```python
from build123d import *

# Parameters (mm, degrees)
BASE_EXTRUDE_DEPTH      = 4.04
BASE_EXTRUDE_DEPTH_BACK = 1.5
SKETCH1_W               = 6.6
SKETCH1_H               = 3.18
SKETCH2_OUTSIDE_W       = 10.436
SKETCH2_OUTSIDE_H       = 7.016
CUT_EXTRUDE1_DEPTH      = 10.990985937
SKETCH3_OUTSIDE_W       = 9.376
SKETCH3_OUTSIDE_H       = 7.016
CUT_EXTRUDE2_DEPTH      = 9.857635125
SKETCH5_W               = 1.63
SKETCH5_H               = 0.38
BOSS_EXTRUDE3_DEPTH     = 0.7
SKETCH6_W               = 0.38
SKETCH6_H               = 1.63
BOSS_EXTRUDE4_DEPTH     = 2.53
SKETCH4_W               = 0.38
SKETCH4_H               = 0.56
BOSS_EXTRUDE5_DEPTH     = 3.28
CUT_EXTRUDE5_DEPTH      = 0.38
FILLET1_R               = 0.49
FILLET2_R               = 0.11
FILLET1_OF_MIRROR1_R    = 0.49
FILLET2_OF_MIRROR1_R    = 0.11
SKETCH10_R              = 0.75
CUT_EXTRUDE6_DEPTH      = 0.7


# Read off the part's stored shape, not the designer's step: Mirror2
with BuildPart() as part:
    # Sketch1 → Base-Extrude (new, two sides: drawn at the far end of the back side and taken through both)
    with BuildSketch(Plane.XY.offset(-BASE_EXTRUDE_DEPTH_BACK)):
        with Locations((3.81, 2.72)):
            Rectangle(SKETCH1_W, SKETCH1_H)
    extrude(amount=BASE_EXTRUDE_DEPTH + BASE_EXTRUDE_DEPTH_BACK)

    # Sketch2 outside → Cut-Extrude1 (cut, through all)
    with BuildSketch(Plane.XY.offset(4.04)):
        with Locations((3.81, 2.72)):
            Rectangle(SKETCH2_OUTSIDE_W, SKETCH2_OUTSIDE_H)
        with BuildLine():
            Line((0.51, 2.91), (0.679431307, 3.748623606))
            ThreePointArc((0.679431307, 3.748623606), (0.922305346, 4.151773257), (1.365567952, 4.31))
            Line((1.365567952, 4.31), (6.254432048, 4.31))
            ThreePointArc((6.254432048, 4.31), (6.697694654, 4.151773257), (6.940568693, 3.748623606))
            Line((6.940568693, 3.748623606), (7.11, 2.91))
            Line((7.11, 2.91), (7.11, 2.53))
            Line((7.11, 2.53), (6.940568693, 1.691376394))
            ThreePointArc((6.940568693, 1.691376394), (6.697694654, 1.288226743), (6.254432048, 1.13))
            Line((6.254432048, 1.13), (1.365567952, 1.13))
            ThreePointArc((1.365567952, 1.13), (0.922305346, 1.288226743), (0.679431307, 1.691376394))
            Line((0.679431307, 1.691376394), (0.51, 2.53))
            Line((0.51, 2.53), (0.51, 2.91))
        make_face(mode=Mode.SUBTRACT)
    extrude(amount=-CUT_EXTRUDE1_DEPTH, mode=Mode.SUBTRACT)

    # Sketch3 outside → Cut-Extrude2 (cut, through all)
    with BuildSketch(Plane(origin=(7.11, 0, 0), x_dir=(0, 0, -1), z_dir=(1, 0, 0))):
        with Locations((-1.27, 2.72)):
            Rectangle(SKETCH3_OUTSIDE_W, SKETCH3_OUTSIDE_H)
        Polygon((1.5, 2.91), (1.134316679, 4.72), (-3.674316679, 4.72), (-4.04, 2.91), (-4.04, 2.53), (-3.674316679, 0.72), (1.134316679, 0.72), (1.5, 2.53), align=None, mode=Mode.SUBTRACT)
    extrude(amount=-CUT_EXTRUDE2_DEPTH, mode=Mode.SUBTRACT)

    # Sketch5 → Boss-Extrude3 (add)
    with BuildSketch(Plane.ZY.offset(-0.51)):
        with Locations((0, 2.72)):
            Rectangle(SKETCH5_W, SKETCH5_H)
    boss_extrude3 = extrude(amount=BOSS_EXTRUDE3_DEPTH)

    # Sketch6 → Boss-Extrude4 (add)
    with BuildSketch(Plane.XZ.offset(-2.53)):
        Rectangle(SKETCH6_W, SKETCH6_H)
    boss_extrude4 = extrude(amount=BOSS_EXTRUDE4_DEPTH)

    # Sketch4 → Boss-Extrude5 (add)
    with BuildSketch(Plane(origin=(0, 0, 0), x_dir=(1, 0, 0), z_dir=(0, 1, 0))):
        Rectangle(SKETCH4_W, SKETCH4_H)
    boss_extrude5 = extrude(amount=-BOSS_EXTRUDE5_DEPTH)

    # Sketch7 → Cut-Extrude5 (cut)
    with BuildSketch(Plane.ZY.offset(0.19)):
        Polygon((0.815, 1.52), (0.55, 0.05), (0.28, 0), (0.28, -3.15), (0.15, -3.28), (-0.15, -3.28), (-0.28, -3.15), (-0.28, 0), (-0.55, 0.05), (-0.815, 1.52), (-0.815, -3.78), (0.815, -3.78), align=None)
    cut_extrude5 = extrude(amount=-CUT_EXTRUDE5_DEPTH, mode=Mode.SUBTRACT)

    # Fillet1
    fillet1_edges = [part.edges().sort_by_distance(p)[0] for p in [
        (-0.19, 2.91, 0),
    ]]
    fillet(fillet1_edges, radius=FILLET1_R)

    # Fillet2
    fillet2_edges = [part.edges().sort_by_distance(p)[0] for p in [
        (0.19, 2.53, 0),
    ]]
    fillet(fillet2_edges, radius=FILLET2_R)

    # Mirror1: Boss-Extrude3, Boss-Extrude4, Boss-Extrude5, Cut-Extrude5 across plane
    add(boss_extrude3.mirror(Plane.ZY.offset(-3.81)))
    add(boss_extrude4.mirror(Plane.ZY.offset(-3.81)))
    add(boss_extrude5.mirror(Plane.ZY.offset(-3.81)))
    add(cut_extrude5.mirror(Plane.ZY.offset(-3.81)), mode=Mode.SUBTRACT)

    # Fillet1 of Mirror1
    fillet1_of_mirror1_edges = [part.edges().sort_by_distance(p)[0] for p in [
        (7.81, 2.91, 0),
    ]]
    fillet(fillet1_of_mirror1_edges, radius=FILLET1_OF_MIRROR1_R)

    # Fillet2 of Mirror1
    fillet2_of_mirror1_edges = [part.edges().sort_by_distance(p)[0] for p in [
        (7.43, 2.53, 0),
    ]]
    fillet(fillet2_of_mirror1_edges, radius=FILLET2_OF_MIRROR1_R)

    # Mirror2: part across plane


with BuildPart() as part_1:
    add(part.part)
    add(part.part.mirror(Plane(origin=(0, 0, 1.27), x_dir=(1, 0, 0), z_dir=(0, 0, -1))))

    # Sketch9 → Cut-Revolve1 (revolve, cut)
    with BuildSketch(Plane.XY):
        with BuildLine():
            Line((2.980337349, 4.31), (2.230337349, 4.31))
            Line((2.230337349, 4.31), (2.230337349, 3.56))
            ThreePointArc((2.230337349, 3.56), (2.760667435, 3.779669914), (2.980337349, 4.31))
        make_face()
    revolve(axis=Axis((2.230337349, 5.149947403, 0), (0, -1, 0)), mode=Mode.SUBTRACT)

    # Sketch10 → Cut-Extrude6 (cut)
    with BuildSketch(Plane(origin=(0, 4.31, 0), x_dir=(-1, 0, 0), z_dir=(0, 1, 0))):
        with Locations((-3.81, -1.5)):
            Circle(SKETCH10_R)
    extrude(amount=-CUT_EXTRUDE6_DEPTH, mode=Mode.SUBTRACT)


solid = part_1.part
```
Part model, mm, in its own coordinate system. A direction names the side the tool comes from. Round coordinates to 2 decimals unless told otherwise and drop trailing zeros. Order: outer loops, then holes, each group sorted by start corner. A loop starts at its lowest first (then second) coordinate and runs counter-clockwise, first axis right, second up. Notation, with made-up numbers: M 5,57.25 L 34,57.25 A3 ccw 34,62.25 Z; hole C -1,-8.5 d8. An arc over 180 degrees is marked long. Answer in a Markdown table with one row per item. Add a question column.
Q1. Cut at B-B on x = 5. Give the cut face in (y, z).
Q2. Pin check, flat tips, straight feed: pin 1 (3 mm diameter, centred on x = 2.5, z = 0, fed in from -Y); pin 2 (0.6 mm diameter, centred on x = 7.5, y = 2, fed in from +Z) (3 decimals). Stop position of each tip, or through.
Q3. Cut at D-D on x = 2.5. Give the cut face in (y, z), and give its area (3 significant figures).
Q4. Mould opens along X. For faces 1 (the face through (4, 4.31, 1)), 2 (the face through (7.026, 2.117, 1.309)), 3 (the face through (0.594, 3.323, 1.309)) say: +X half, -X half, draft (parallel to the pull), parting line (faces both ways), or undercut.
Q5. Cut at A-A on y = -1.75. Give the cut face in (x, z), and give its area (3 significant figures).
Q6. 3-axis set-ups, long thin cutter, end or side, ignore diameter. For faces 4 (the face through (0.19, 0.2, 2.6)), 5 (the face through (3.86, 1.84, 3.9)): which of +Z, -Z, +X, -X, +Y, -Y reach the whole face in a straight line?
Q7. Cut at C-C on z = 3.6. Give the cut face in (x, y).
Q8. Wall check: L1, parallel to X at y = -2.75, z = 0.05; L2, parallel to X at y = 2.25, z = -0.65; L3, parallel to Y at x = 3.25, z = 1.6. Give the ranges that are in metal, low to high. Write a range as from..to.
Established:
| question | item | result |
|---|---|---|
| 1 | outline | M 1.13,-1.22 L 2.53,-1.5 L 2.91,-1.5 L 4.31,-1.22 L 4.31,3.76 L 2.91,4.04 L 2.53,4.04 L 1.13,3.76 Z |
| 2 | pin 1 | stops at y = 1.13 |
| 2 | pin 2 | stops at z = 3.355 |
| 3 | outline | M 1.13,-1.22 L 2.53,-1.5 L 2.91,-1.5 L 4.31,-1.22 L 4.31,-0.7 A0.7 cw 4.31,0.7 L 4.31,3.76 L 2.91,4.04 L 2.53,4.04 L 1.13,3.76 Z |
| 3 | area | 16.1 mm2 |
| 4 | face 1 | draft |
| 4 | face 2 | undercut |
| 4 | face 3 | -X half |
| 5 | outline | M -0.19,-0.28 L 0.19,-0.28 L 0.19,0.28 L -0.19,0.28 Z; M -0.19,2.26 L 0.19,2.26 L 0.19,2.82 L -0.19,2.82 Z; M 7.43,-0.28 L 7.81,-0.28 L 7.81,0.28 L 7.43,0.28 Z; M 7.43,2.26 L 7.81,2.26 L 7.81,2.82 L 7.43,2.82 Z |
| 5 | area | 0.851 mm2 |
| 6 | face 4 | +Z, -Z, -Y |
| 6 | face 5 | +Z, +X, -X, -Y |
| 7 | outline | M 0.51,2.53 L 0.68,1.69 A0.7 ccw 1.37,1.13 L 6.25,1.13 A0.7 ccw 6.94,1.69 L 7.11,2.53 L 7.11,2.91 L 6.94,3.75 A0.7 ccw 6.25,4.31 L 1.37,4.31 A0.7 ccw 0.68,3.75 L 0.51,2.91 Z |
| 8 | L1 | x = -0.19..0.19, 7.43..7.81 |
| 8 | L2 | x = -0.19..0.19, 0.57..7.05, 7.43..7.81 |
| 8 | L3 | y = 1.13..4.31 |
